Solid Edge part; units mm, degrees
sketch "Sketch1" plane through (0, 0, 0) normal (0, 0, 1) x (1, 0, 0)
  line L0 (75, -50) -> (75, 50)
  line L1 (75, 50) -> (-75, 50)
  line L2 (-75, 50) -> (-75, -50)
  line L3 (-75, -50) -> (75, -50)
extrude "Protrusion1" add sketch "Sketch1" against normal blind 15
sketch "Sketch2" plane through (0, 0, 0) normal (0, 0, 1) x (1, 0, 0)
  circle A0 centre (0, 0) radius 33
extrude "ExtrudedProtrusion_2" add sketch "Sketch2" along normal blind 50
sketch "Sketch3" plane through (0, 0, 50) normal (0, 0, 1) x (1, 0, 0)
  arc A0 (-55.2632, 12.1692) -> (55.2632, 12.1692) centre (0, -38.5357) cw
  arc A1 (55.2632, -12.1692) -> (55.2632, 12.1692) centre (42, 0) ccw
  arc A2 (-55.2632, -12.1692) -> (55.2632, -12.1692) centre (0, 38.5357) ccw
  arc A3 (-55.2632, 12.1692) -> (-55.2632, -12.1692) centre (-42, 0) ccw
extrude "ExtrudedProtrusion_3" add sketch "Sketch3" along normal blind 15
sketch "Sketch4" plane through (0, 0, 0) normal (0, -1, 0) x (1, 0, 0)
  line L0 (21, 65) -> (21, 0)
  line L1 (21, 0) -> (16.5, 0)
  line L2 (16.5, -15) -> (16.5, 0)
  line L3 (0, -15) -> (16.5, -15)
  line L4 (0, -15) -> (0, 65)
  line L5 (0, 65) -> (21, 65)
revolve "RevolvedCutout1" cut sketch "Sketch4" angle 360 about axis through (0, 0, -15) along (0, 0, 1)
sketch "Sketch5" plane through (0, 0, 65) normal (0, 0, 1) x (1, 0, 0)
  circle A0 centre (42, 0) radius 6
  circle A1 centre (-42, 0) radius 6
extrude "ExtrudedCutout_1" cut sketch "Sketch5" against normal blind 15
properties material "StCst10 GOST 1412-85"
For this review, take the finished solid that the model builds, in its own axes (mm). A direction names the side the tool comes from. Round coordinates to 2 decimals unless told otherwise and drop trailing zeros. Write each loop counter-clockwise with the first axis right and the second up, starting at its lowest first coordinate (ties: lowest second). Pieces come first, ordered by that corner, then holes. Notation, with made-up numbers: (-25, -21.5) - (14, -21.5) arc R15 cw to (14, 2.5) - close; hole circle Ø7 at (-8.5, -5). An arc over 180 degrees is marked (long way). Answer as CSV lines item,"result". Start each with the question number.
(1) Add section C-C, the plane z = -4.5. State the section outline as (x, y) points.
(2) Add section D-D, the plane x = 42. State the section outline as (y, z) points.
(3) Mouldability with a two-part tool opening along Z and no side actions: class faces 1 (the flat face through (9, -32, 50)), 2 (the flat face through (-1, -50, -7)), 3 (the flat face through (-18, 1, -15)) as +Z half, -Z half, draft (parallel to the pull), parting line (faces both ways), or undercut.
(4) For pin 1 (12 mm diameter, centred on x = -53, z = 56, fed in from -Y); pin 2 (21 mm diameter, centred on x = 1, y = 9.5, fed in from +Z); pin 3 (8 mm diameter, centred on y = -14, z = 6.5, fed in from +X); pin 4 (19 mm diameter, centred on x = 42, y = 0, fed in from +Z), all flat-tipped, find the tip position at first contact; note any pin that passes through.
(5) For line 1 (Z direction, x = 33.5, y = 6.5); line 2 (Y direction, x = 0, z = 42.5); line 3 (Y direction, x = 0, z = -5.5), list the stretches that pass through material, from the lowest coordinate up.
(6) Add section B-B, the plane y = 0. State the section outline as (x, z) points, plus the area to 4 significant figures.
(7) Add section A-A, the plane x = 0. State the section outline as (y, z) points.
(8) Machinability: for faces 4 (the cylindrical face through (0.87, -36.46, 57.4)), 5 (the cylindrical face through (30.5, 12.6, 24.6)), 6 (the cylindrical face through (60, 0, 57)), 7 (the cylindrical face through (-0.87, 36.46, 57.4)), 8 (the cylindrical face through (20.03, -6.31, 32.04)), which of the approach directions +Z, -Z, +X, -X, +Y, -Y give a long, thin tool a straight path to every point of the face, cutting with its end or side? Answer none if there is none.
From the geometry:
1,outline,"(-75, -50) - (75, -50) - (75, 50) - (-75, 50) - close; hole circle Ø33 at (0, 0)"
2,outline,"(-50, -15) - (50, -15) - (50, 0) - (-50, 0) - close; (-23.6, 50) - (-6, 50) - (-6, 65) - (-23.6, 65) - close; (6, 50) - (23.6, 50) - (23.6, 65) - (6, 65) - close"
3,face 1,"undercut"
3,face 2,"draft"
3,face 3,"-Z half"
4,pin 1,"stops at y = -19.91"
4,pin 2,"stops at z = 0"
4,pin 3,"stops at x = 31.45"
4,pin 4,"stops at z = 65"
5,line 1,"z = -15 to 0, 50 to 65"
5,line 2,"y = -33 to -21, 21 to 33"
5,line 3,"y = -50 to -16.5, 16.5 to 50"
6,outline,"(-75, -15) - (-16.5, -15) - (-16.5, 0) - (-21, 0) - (-21, 65) - (-36, 65) - (-36, 50) - (-33, 50) - (-33, 0) - (-75, 0) - close; (-60, 50) - (-48, 50) - (-48, 65) - (-60, 65) - close; (16.5, -15) - (75, -15) - (75, 0) - (33, 0) - (33, 50) - (36, 50) - (36, 65) - (21, 65) - (21, 0) - (16.5, 0) - close; (48, 50) - (60, 50) - (60, 65) - (48, 65) - close"
6,area,"3,765 mm²"
7,outline,"(-50, -15) - (-16.5, -15) - (-16.5, 0) - (-21, 0) - (-21, 65) - (-36.46, 65) - (-36.46, 50) - (-33, 50) - (-33, 0) - (-50, 0) - close; (16.5, -15) - (50, -15) - (50, 0) - (33, 0) - (33, 50) - (36.46, 50) - (36.46, 65) - (21, 65) - (21, 0) - (16.5, 0) - close"
8,face 4,"+Z, -Y"
8,face 5,"none"
8,face 6,"+Z, +X"
8,face 7,"+Z, +Y"
8,face 8,"+Z"
